The model under review builds one solid part; all positions refer to its coordinate system, in mm. A direction names the side the tool comes from. Coordinates: 2 decimals unless noted, no trailing zeros. Order: outer loops, then holes, each group sorted by start corner. A loop starts at its lowest first (then second) coordinate and runs counter-clockwise, first axis right, second up.
```python
from build123d import *

# Parameters (mm, degrees)
BOSS_EXTRU_1_DEPTH = 5
BOSS_EXTRU_2_START = -5
ESQUISSE2_W        = 208.80895352
ESQUISSE2_H        = 208.80895352
ESQUISSE2_R        = 87.5
ESQUISSE2_R_2      = 1.5
ESQUISSE2_W_2      = 5
ESQUISSE2_H_2      = 5
BOSS_EXTRU_2_DEPTH = 5


# Read off the part's stored shape, not the designer's step: Boss.-Extru.1
with BuildPart() as part:
    # Boss.-Extru.1 outline → Boss.-Extru.1 (new body)
    with BuildSketch(Plane.XY):
        with BuildLine():
            Line((-15, 94.40447676), (-15, 99.40447676))
            Line((-15, 99.40447676), (-25, 99.40447676))
            ThreePointArc((-25, 99.40447676), (-72.478445072, 72.478445072), (-99.40447676, 25))
            Line((-99.40447676, 25), (-99.40447676, 15))
            Line((-99.40447676, 15), (-94.40447676, 15))
            Line((-94.40447676, 15), (-94.40447676, -15))
            Line((-94.40447676, -15), (-99.40447676, -15))
            Line((-99.40447676, -15), (-99.40447676, -25))
            ThreePointArc((-99.40447676, -25), (-72.478445072, -72.478445072), (-25, -99.40447676))
            Line((-25, -99.40447676), (-15, -99.40447676))
            Line((-15, -99.40447676), (-15, -94.40447676))
            Line((-15, -94.40447676), (15, -94.40447676))
            Line((15, -94.40447676), (15, -99.40447676))
            Line((15, -99.40447676), (25, -99.40447676))
            ThreePointArc((25, -99.40447676), (72.478445072, -72.478445072), (99.40447676, -25))
            Line((99.40447676, -25), (99.40447676, -15))
            Line((99.40447676, -15), (94.40447676, -15))
            Line((94.40447676, -15), (94.40447676, 15))
            Line((94.40447676, 15), (99.40447676, 15))
            Line((99.40447676, 15), (99.40447676, 25))
            ThreePointArc((99.40447676, 25), (72.478445072, 72.478445072), (25, 99.40447676))
            Line((25, 99.40447676), (15, 99.40447676))
            Line((15, 99.40447676), (15, 94.40447676))
            Line((15, 94.40447676), (-15, 94.40447676))
        make_face()
        with BuildLine():
            ThreePointArc((-2.061552813, -83.5), (-3.811893422, -85.108458961), (-4.498511999, -87.384285714))
            ThreePointArc((-4.498511999, -87.384285714), (-61.871843354, -61.871843354), (-87.384285714, -4.498511999))
            ThreePointArc((-87.384285714, -4.498511999), (-85.108458961, -3.811893422), (-83.5, -2.061552813))
            Line((-83.5, -2.061552813), (-83.5, 2.061552813))
            ThreePointArc((-83.5, 2.061552813), (-85.108458961, 3.811893422), (-87.384285714, 4.498511999))
            ThreePointArc((-87.384285714, 4.498511999), (-61.871843354, 61.871843354), (-4.498511999, 87.384285714))
            ThreePointArc((-4.498511999, 87.384285714), (-3.811893422, 85.108458961), (-2.061552813, 83.5))
            Line((-2.061552813, 83.5), (2.061552813, 83.5))
            ThreePointArc((2.061552813, 83.5), (3.811893422, 85.108458961), (4.498511999, 87.384285714))
            ThreePointArc((4.498511999, 87.384285714), (61.871843354, 61.871843354), (87.384285714, 4.498511999))
            ThreePointArc((87.384285714, 4.498511999), (85.108458961, 3.811893422), (83.5, 2.061552813))
            Line((83.5, 2.061552813), (83.5, -2.061552813))
            ThreePointArc((83.5, -2.061552813), (85.108458961, -3.811893422), (87.384285714, -4.498511999))
            ThreePointArc((87.384285714, -4.498511999), (61.871843354, -61.871843354), (4.498511999, -87.384285714))
            ThreePointArc((4.498511999, -87.384285714), (3.811893422, -85.108458961), (2.061552813, -83.5))
            Line((2.061552813, -83.5), (-2.061552813, -83.5))
        make_face(mode=Mode.SUBTRACT)
    extrude(amount=BOSS_EXTRU_1_DEPTH)

    # Esquisse2 → Boss.-Extru.2 (add)
    with BuildSketch(Plane.XY.offset(5).offset(BOSS_EXTRU_2_START)):
        Rectangle(ESQUISSE2_W, ESQUISSE2_H)
        Circle(ESQUISSE2_R, mode=Mode.SUBTRACT)
        with Locations((0, 96.90447676)):
            Circle(ESQUISSE2_R_2, mode=Mode.SUBTRACT)
        with Locations((96.90447676, 0)):
            Circle(ESQUISSE2_R_2, mode=Mode.SUBTRACT)
        with Locations((0, -96.90447676)):
            Circle(ESQUISSE2_R_2, mode=Mode.SUBTRACT)
        with Locations((-96.90447676, 0)):
            Circle(ESQUISSE2_R_2, mode=Mode.SUBTRACT)
        with Locations((-7.5, 96.90447676)):
            Rectangle(ESQUISSE2_W_2, ESQUISSE2_H_2, mode=Mode.SUBTRACT)
        with Locations((7.5, 96.90447676)):
            Rectangle(ESQUISSE2_W_2, ESQUISSE2_H_2, mode=Mode.SUBTRACT)
        with Locations((96.90447676, 7.5)):
            Rectangle(ESQUISSE2_W_2, ESQUISSE2_H_2, mode=Mode.SUBTRACT)
        with Locations((96.90447676, -7.5)):
            Rectangle(ESQUISSE2_W_2, ESQUISSE2_H_2, mode=Mode.SUBTRACT)
        with Locations((7.5, -96.90447676)):
            Rectangle(ESQUISSE2_W_2, ESQUISSE2_H_2, mode=Mode.SUBTRACT)
        with Locations((-7.5, -96.90447676)):
            Rectangle(ESQUISSE2_W_2, ESQUISSE2_H_2, mode=Mode.SUBTRACT)
        with Locations((-96.90447676, -7.5)):
            Rectangle(ESQUISSE2_W_2, ESQUISSE2_H_2, mode=Mode.SUBTRACT)
        with Locations((-96.90447676, 7.5)):
            Rectangle(ESQUISSE2_W_2, ESQUISSE2_H_2, mode=Mode.SUBTRACT)
    extrude(amount=BOSS_EXTRU_2_DEPTH)


solid = part.part
```
(1) Draft analysis for pull direction X (two halves, no side actions). For faces 3 (the face through (91, 1, 5)), 4 (the face through (-8, 99.404, 2)), state which applies: released by +X, released by -X, zero draft, split by the parting line, or undercut.
A:
face 3: zero draft
face 4: undercut
(2) We need section C-C, the plane z = 2.85. Count the separate pieces of the cut face and the enclosed holes in it, and give its area (3 significant figures).
A:
separate pieces: 1
enclosed holes: 13
area: 19,400 mm2
(3) We need section B-B, the plane x = -79.5. Write out the cut boundary in (y, z).
A:
outline: (-104.4, 0) - (-36.55, 0) - (-36.55, 5) - (-104.4, 5) - close; (36.55, 0) - (104.4, 0) - (104.4, 5) - (36.55, 5) - close
(4) Machinability: for faces 1 (the face through (91, 1, 0)), 2 (the face through (5, -97, 2)), which of the approach directions +Z, -Z, +X, -X, +Y, -Y give a long, thin tool a straight path to every point of the face, cutting with its end or side? Answer none if there is none.
A:
face 1: -Z, +X, -X, +Y, -Y
face 2: +Z, -Z
(5) Wall thickness on probe 1 along Y at (x, z) = (0, 3.95); probe 2 along X at (y, z) = (-14.5, 1.65); probe 3 along Y at (x, z) = (-17.5, 4.3): over which ranges is each line inside the solid? List them lowest first.
A:
probe 1: y = -104.4 to -98.4, -95.4 to -83.5, 83.5 to 95.4, 98.4 to 104.4
probe 2: x = -104.4 to -86.29, 86.29 to 104.4
probe 3: y = -104.4 to -85.73, 85.73 to 104.4
(6) We need section A-A, the plane y = -29. Write out the cut boundary in (x, z).
A:
outline: (-104.4, 0) - (-82.55, 0) - (-82.55, 5) - (-104.4, 5) - close; (82.55, 0) - (104.4, 0) - (104.4, 5) - (82.55, 5) - close
